Autodesk Inventor part; units mm, degrees
ref_plane "YZ Plane" through (0, 0, 0) normal (1, 0, 0) x (0, 1, 0)
ref_plane "XZ Plane" through (0, 0, 0) normal (0, 1, 0) x (-1, 0, 0)
ref_plane "XY Plane" through (0, 0, 0) normal (0, 0, 1) x (1, 0, 0)
sketch "Sketch1" plane through (0, 0, 0) normal (0, 1, 0) x (-1, 0, 0)
  line L0 (0, 0) -> (0, -3)
  line L1 (0, -3) -> (-2.5981, -1.5)
  line L2 (-2.5981, -1.5) -> (-2.5981, 1.5)
  line L3 (-2.5981, 1.5) -> (0, 3)
  line L4 (0, 3) -> (2.5981, 1.5)
  line L5 (2.5981, 1.5) -> (2.5981, -1.5)
  line L6 (2.5981, -1.5) -> (0, -3)
  dimension "d0" = 3
extrude "Extrusion1" add sketch "Sketch1" along normal blind 10
sketch "Sketch2" plane through (0, 10, 0) normal (0, 1, 0) x (1, 0, 0)
  point P0 (0, 0)
  point P1 (0, 0)
hole "Hole1" at (0, 10, 0) direction (0, -1, 0) diameter 3.2 end through all
properties part number "M3x10-threaded"
The listing builds one solid part. Answer for the finished solid, in the listing's coordinates (mm). Give positions to 0.01 mm unless a question says otherwise; leave off trailing zeros. Order: outer loops, then holes, each group sorted by start corner. A loop starts at its lowest first (then second) coordinate and runs counter-clockwise, first axis right, second up. Notation, with made-up numbers: (55.5, 88.5) - (98.5, 88.5) arc R36 ccw to (98.5, 125.5) - close; hole circle Ø11 at (-29, 36.25). An arc over 180 degrees is marked (long way). Answer in a Markdown table with one row per item. Add a question column.
Q1. The part is cut by section A-A (y = 2.5). Determine the outline of the cut face in (x, z), then the cut area to 3 significant figures.
Q2. Find the intervals of material crossed by line 1 along X through (y, z) = (7.25, 0); line 2 along Z through (x, y) = (0.7, 6.75); line 3 along Z through (x, y) = (-1.2, 6.25), in increasing order. Write a range as [from, to].
Q3. The part is cut by section B-B (z = 0). Determine the outline of the cut face in (x, y), then the cut area to 3 significant figures.
Q4. The part is cut by section C-C (x = -0.8). Determine the outline of the cut face in (y, z), then the cut area to 3 significant figures.
Q5. The part is cut by section D-D (x = 1.95). Determine the outline of the cut face in (y, z), then the cut area to 3 significant figures.
Q6. Given P1, Ø2, axis at x = 0.5, y = 5.5, coming from the +Z side, flat-ended and moving along its own axis, determine where the tip first touches the part or whether it passes through.
Q7. For a pull along X with two mould halves and no side action, classify faces 1 (the cylindrical face through (0.97, 4.93, -1.27)), 2 (the flat face through (1.2, 10, -1.3)), 3 (the flat face through (-2.598, 5, 0)) as released by +X, released by -X, zero draft, split by the parting line, or undercut.
Determined:
| question | item | result |
|---|---|---|
| 1 | outline | (-2.6, -1.5) - (0, -3) - (2.6, -1.5) - (2.6, 1.5) - (0, 3) - (-2.6, 1.5) - close; hole circle Ø3.2 at (0, 0) |
| 1 | area | 15.3 mm² |
| 2 | line 1 | x = [-2.6, -1.6], [1.6, 2.6] |
| 2 | line 2 | z = [-2.6, -1.44], [1.44, 2.6] |
| 2 | line 3 | z = [-2.31, -1.06], [1.06, 2.31] |
| 3 | outline | (-2.6, 0) - (-1.6, 0) - (-1.6, 10) - (-2.6, 10) - close; (1.6, 0) - (2.6, 0) - (2.6, 10) - (1.6, 10) - close |
| 3 | area | 20.0 mm² |
| 4 | outline | (0, -2.54) - (10, -2.54) - (10, -1.39) - (0, -1.39) - close; (0, 1.39) - (10, 1.39) - (10, 2.54) - (0, 2.54) - close |
| 4 | area | 23.0 mm² |
| 5 | outline | (0, -1.87) - (10, -1.87) - (10, 1.87) - (0, 1.87) - close |
| 5 | area | 37.5 mm² |
| 6 | P1 | stops at z = 3 |
| 7 | face 1 | undercut |
| 7 | face 2 | zero draft |
| 7 | face 3 | released by -X |
